The model under review builds one solid part; all positions refer to its coordinate system, in mm. Face numbers are marked on the shaded views. A direction names the side the tool comes from. Give positions to 0.01 mm unless a question says otherwise; leave off trailing zeros. Order: outer loops, then holes, each group sorted by start corner. A loop starts at its lowest first (then second) coordinate and runs counter-clockwise, first axis right, second up. Notation, with made-up numbers: (54.25, 13.5) - (62.25, 13.5) arc R34 ccw to (62.25, 52.5) - close; hole circle Ø7 at (-4, 29.5). An arc over 180 degrees is marked (long way). Use a Markdown table: item, result. Add a question column.
```python
from build123d import *

# Parameters (mm, degrees)
F1_DEPTH = 800
F2_W     = 152.4
F2_H     = 152.4
F3_DEPTH = 4.7625
F4_W     = 152.4
F4_H     = 804.7625
F5_DEPTH = 4.7625
F6_W     = 152.4
F6_H     = 150
F7_DEPTH = 1.21
F9_DEPTH = 71.464


# Not quite as in the source:
# - a length typed as a fraction of an inch, garbled in the dataset ("3 / 203.2 mm" for 3/8 in), is restored


with BuildPart() as f1:
    # F0 (on Top) → F1 (new body)
    with BuildSketch(Plane.XY):
        Polygon((-76.2, 76.2), (-76.2, -76.2), (-71.437, -76.2), (-71.437, -2.3815), (71.437, -2.3815), (71.437, -76.2), (76.2, -76.2), (76.2, 76.2), (71.437, 76.2), (71.437, 2.382), (-71.437, 2.382), (-71.437, 76.2), align=None)
    extrude(amount=-F1_DEPTH)

    # F2 (on face) → F3 (join)
    with BuildSketch(Plane.XY):
        Rectangle(F2_W, F2_H)
    extrude(amount=F3_DEPTH)

    # F4 (on face) → F5 (join)
    with BuildSketch(Plane(origin=(0, 76.2, 0), x_dir=(-1, 0, 0), z_dir=(0, 1, 0))):
        with Locations((0, -397.61875)):
            Rectangle(F4_W, F4_H)
    extrude(amount=F5_DEPTH)

    # F6 (on face) → F7 (join)
    with BuildSketch(Plane.XZ.offset(76.2)):
        with Locations((0, -70.2375)):
            Rectangle(F6_W, F6_H)
    extrude(amount=F7_DEPTH)

    # F8 (on Right) → F9 (join, symmetric)
    with BuildSketch(Plane.YZ):
        Polygon((-76.13632828, -800.0091910362), (-74.92632828, -800.0091910362), (0.8852251628, 4.7220308334), (-0.3247748372, 4.7220308334), align=None)
    extrude(amount=F9_DEPTH, both=True)


solid = f1.part
```
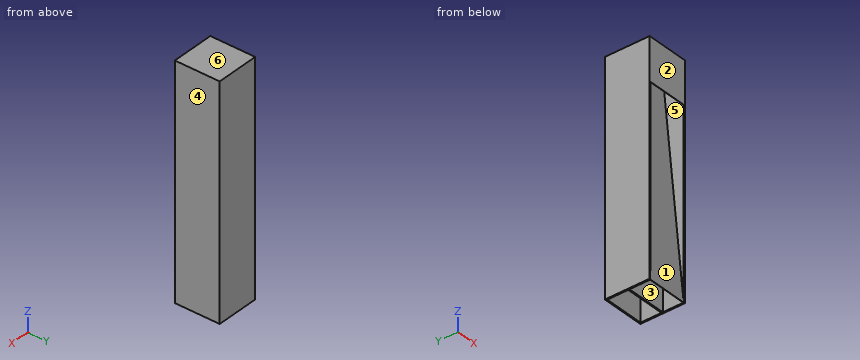
Q1. Clearance check with flat-ended pins moving along their axes: P1, Ø1, axis at x = 58, z = -212, coming from the -Y side; P2, Ø1.5, axis at x = -1.5, z = -545.5, coming from the -Y side; P3, Ø4, axis at x = 74, z = -623, coming from the -Y side. State where each tip first meets the part, or that it passes through.
Q2. Draft analysis for pull direction Z (two halves, no side actions). For the marked faces 4, 5 and 6, state which applies: pulls with the +Z half, pulls with the -Z half, needs draft (parallel to the pull), parting line crosses it, or undercut.
Q3. We need section A-A (y = 62). Write out the cut boundary in (x, z), plus the area to 3 significant figures.
Q4. Machinability: for the marked faces 1, 2 and 3, which of the approach directions +Z, -Z, +X, -X, +Y, -Y give a long, thin tool a straight path to every point of the face, cutting with its end or side? Answer none if there is none.
Q5. We need section B-B (z = -367). Write out the cut boundary in (x, y), plus the area to 3 significant figures.
Q6. We need section C-C (x = 32.5). Write out the cut boundary in (y, z).
Q7. Wall thickness on probe 1 along X at (y, z) = (37.5, -115); probe 2 along Y at (x, z) = (-14.5, -493.5); probe 3 along Y at (x, z) = (20.5, -392.5): over which ranges is each line inside the solid? List them lowest first.
Q8. We need section D-D (z = -134.5). Write out the cut boundary in (x, y).
Here are the results:
| question | item | result |
|---|---|---|
| 1 | P1 | y = -20.79 |
| 1 | P2 | y = -52.23 |
| 1 | P3 | y = -76.2 |
| 2 | face 4 | needs draft |
| 2 | face 5 | undercut |
| 2 | face 6 | pulls with the +Z half |
| 3 | outline | (-76.2, -800) - (-71.44, -800) - (-71.44, 0) - (71.44, 0) - (71.44, -800) - (76.2, -800) - (76.2, 4.76) - (-76.2, 4.76) - close |
| 3 | area | 8,350 mm2 |
| 4 | face 1 | none |
| 4 | face 2 | +Z, -Z, +X, -X, -Y |
| 4 | face 3 | -Z |
| 5 | outline | (-76.2, -76.2) - (-71.44, -76.2) - (-71.44, -35.34) - (71.44, -35.34) - (71.44, -76.2) - (76.2, -76.2) - (76.2, 80.96) - (-76.2, 80.96) - close; hole (-71.44, -34.13) - (71.44, -34.13) - (71.44, -2.38) - (-71.44, -2.38) - close; hole (-71.44, 2.38) - (71.44, 2.38) - (71.44, 76.2) - (-71.44, 76.2) - close |
| 5 | area | 3,030 mm2 |
| 6 | outline | (-77.41, -145.24) - (-76.2, -145.24) - (-76.2, 0) - (-2.38, 0) - (-2.38, -17.11) - (-76.14, -800.01) - (-74.93, -800.01) - (-2.38, -29.95) - (-2.38, -800) - (2.38, -800) - (2.38, 0) - (76.2, 0) - (76.2, -800) - (80.96, -800) - (80.96, 4.76) - (-77.41, 4.76) - close |
| 7 | probe 1 | -76.2 to -71.44, 71.44 to 76.2 |
| 7 | probe 2 | -47.26 to -46.05, -2.38 to 2.38, 76.2 to 80.96 |
| 7 | probe 3 | -37.75 to -36.54, -2.38 to 2.38, 76.2 to 80.96 |
| 8 | outline | (-76.2, -77.41) - (76.2, -77.41) - (76.2, 80.96) - (-76.2, 80.96) - close; hole (-71.44, -76.2) - (71.44, -76.2) - (71.44, -13.44) - (-71.44, -13.44) - close; hole (-71.44, -12.23) - (71.44, -12.23) - (71.44, -2.38) - (-71.44, -2.38) - close; hole (-71.44, 2.38) - (71.44, 2.38) - (71.44, 76.2) - (-71.44, 76.2) - close |
